Read the model definition and answer for the solid it produces. Units are mm, in the model's axes. Face numbers are marked on the shaded views. A direction names the side the tool comes from. Coordinates: 2 decimals unless noted, no trailing zeros. Write each loop counter-clockwise with the first axis right and the second up, starting at its lowest first coordinate (ties: lowest second). Pieces come first, ordered by that corner, then holes.
Item 1: Section B-B (z = 10.25) is taken. Give the vertices of the cut face in (x, y).
Item 2: A tool of negligible diameter and unlimited length cuts with its end or side. For the marked faces 1 and 2, from which of +Z, -Z, +X, -X, +Y, -Y can it reach the whole face along a straight path? Write none if from no direction.
Item 3: Each of these flat-tipped pins is pushed along its axis until it touches: P1, Ø8, axis at x = 26.5, y = -1, coming from the -Z side; P2, Ø1.4, axis at y = 0, z = 3.5, coming from the +X side; P3, Ø8, axis at x = 11.5, y = 0, coming from the +Z side; P4, Ø1.5, axis at x = 39, y = -10, coming from the +Z side. Where does it stop, or does it pass through?
Item 4: Determine the mould class of the marked faces 3, 4, 5 and 6 for opening direction Y: released by +Y, released by -Y, zero draft, split by the parting line, or undercut.
Item 5: Section A-A (y = 0) is taken. Give the vertices of the cut face in (x, z).
Item 6: Section D-D (x = -7) is taken. Give the vertices of the cut face in (y, z).
Item 7: Straight lines are drawn through the part: probe 1 along X at (y, z) = (3, 9.5); probe 2 along Y at (x, z) = (115.5, 9.25); probe 3 along Y at (x, z) = (111, 3.25). For each, find the intervals that lie inside material, in ascending order.
Item 8: Section C-C (x = 105) is taken. Give the vertices of the cut face in (y, z), then the cut area to 3 significant figures.
from build123d import *

# Parameters (mm, degrees)
F0_W         = 50.5
F0_H         = 9
F0_H_2       = 2
F0_W_2       = 12.75
F0_H_3       = 0.25
F0_W_3       = 1.2480659857
F1_DEPTH     = 1.5
F0_W_4       = 77.7519340143
F2_DEPTH     = 6.5
F3_DEPTH     = 15
F4_R         = 2
F5_DEPTH     = 162.001
F6_R         = 2
F7_T1_DEPTH  = 27.5
F7_T4_ANGLE  = 90
F7_T6_ANGLE  = 90
F7_T8_ANGLE  = 90
F7_T10_ANGLE = 90


# Not quite as in the source:
# - a fillet or chamfer that OpenCascade refuses, or shapes differently, is made with other operations: its cross-section is extruded or revolved along the edge and cut away or added


with BuildPart() as f1:
    # F0 (on Top) → F1 (new body)
    with BuildSketch(Plane.XY):
        with Locations((8.0849453807, 6.5)):
            Rectangle(F0_W, F0_H)
        with Locations((8.0849453807, 1)):
            Rectangle(F0_W, F0_H_2)
        with Locations((8.0849453807, -1)):
            Rectangle(F0_W, F0_H_2)
        with Locations((-23.5400546193, -1)):
            Rectangle(F0_W_2, F0_H_2)
        with Locations((-23.5400546193, 1)):
            Rectangle(F0_W_2, F0_H_2)
        with Locations((39.7099453807, 1)):
            Rectangle(F0_W_2, F0_H_2)
        with Locations((39.7099453807, -1)):
            Rectangle(F0_W_2, F0_H_2)
        Polygon((46.0849453807, 2), (46.0849453807, 0), (46.0849453807, -2), (123.8368793949, -2), (123.8368793949, 2), align=None)
        with Locations((8.0849453807, -6.5)):
            Rectangle(F0_W, F0_H)
        with Locations((8.0849453807, 11.125)):
            Rectangle(F0_W, F0_H_3)
        with Locations((8.0849453807, -11.125)):
            Rectangle(F0_W, F0_H_3)
        with Locations((-30.5390876122, -1)):
            Rectangle(F0_W_3, F0_H_2)
        with Locations((-30.5390876122, 1)):
            Rectangle(F0_W_3, F0_H_2)
    extrude(amount=F1_DEPTH)

    # F0 (on Top) → F2 (join)
    with BuildSketch(Plane.XY):
        with Locations((-23.5400546193, 6.5)):
            Rectangle(F0_W_2, F0_H)
        with Locations((-30.5390876122, 6.5)):
            Rectangle(F0_W_3, F0_H)
        with Locations((-23.5400546193, -6.5)):
            Rectangle(F0_W_2, F0_H)
        with Locations((-30.5390876122, -6.5)):
            Rectangle(F0_W_3, F0_H)
        with Locations((39.7099453807, -6.5)):
            Rectangle(F0_W_2, F0_H)
        with Locations((39.7099453807, 6.5)):
            Rectangle(F0_W_2, F0_H)
        with Locations((84.9609123878, 6.5)):
            Rectangle(F0_W_4, F0_H)
        with Locations((84.9609123878, -6.5)):
            Rectangle(F0_W_4, F0_H)
    extrude(amount=F2_DEPTH)

    # F0 (on Top) → F3 (join)
    with BuildSketch(Plane.XY):
        Polygon((127.3368793949, -15), (127.3368793949, 15), (-34.6631206051, 15), (-34.6631206051, 0), (-34.6631206051, -15), align=None)
        Polygon((-31.1631206051, -2), (-31.1631206051, 0), (-31.1631206051, 2), (-31.1631206051, 11), (-29.9150546193, 11), (-17.1650546193, 11), (-17.1650546193, 11.25), (33.3349453807, 11.25), (33.3349453807, 11), (46.0849453807, 11), (123.8368793949, 11), (123.8368793949, 2), (123.8368793949, -2), (123.8368793949, -11), (46.0849453807, -11), (33.3349453807, -11), (33.3349453807, -11.25), (-17.1650546193, -11.25), (-17.1650546193, -11), (-29.9150546193, -11), (-31.1631206051, -11), align=None, mode=Mode.SUBTRACT)
    extrude(amount=F3_DEPTH)

    # F4 (on face) → F5 (cut, through all)
    with BuildSketch(Plane.YZ.offset(127.3368793949)):
        with Locations((0, 4.3932246044)):
            Circle(F4_R)
    extrude(amount=-F5_DEPTH, mode=Mode.SUBTRACT)

    # F6
    f6_edges = [f1.edges().sort_by_distance(p)[0] for p in [
        (-24.164088, -2, 6.5),
        (-24.164088, 2, 6.5),
        (-17.165055, -6.5, 6.5),
        (-17.165055, 6.5, 6.5),
        (33.334945, 6.5, 6.5),
        (33.334945, -6.5, 6.5),
        (78.585912, -2, 6.5),
        (78.585912, 2, 6.5),
        (46.336879, 15, 15),
        (-34.663121, 0, 15),
        (46.336879, -15, 15),
        (127.336879, 0, 15),
    ]]
    fillet(f6_edges, radius=F6_R)

    # F7: fillet of radius 5 on 4 edges, made by hand

    # F7_s2 → F7_t1 (cut)
    with BuildSketch(Plane.XY.offset(-12.5)):
        with BuildLine():
            ThreePointArc((-29.6631206051, 15), (-33.198654511, 13.5355339059), (-34.6631206051, 10))
            Line((-34.6631206051, 10), (-34.6631206051, 15))
            Line((-34.6631206051, 15), (-29.6631206051, 15))
        make_face()
        with BuildLine():
            ThreePointArc((-34.6631206051, -10), (-33.198654511, -13.5355339059), (-29.6631206051, -15))
            Line((-29.6631206051, -15), (-34.6631206051, -15))
            Line((-34.6631206051, -15), (-34.6631206051, -10))
        make_face()
        with BuildLine():
            ThreePointArc((122.3368793949, 15), (125.8724133009, 13.5355339059), (127.3368793949, 10))
            Line((127.3368793949, 10), (127.3368793949, 15))
            Line((127.3368793949, 15), (122.3368793949, 15))
        make_face()
        with BuildLine():
            ThreePointArc((127.3368793949, -10), (125.8724133009, -13.5355339059), (122.3368793949, -15))
            Line((122.3368793949, -15), (127.3368793949, -15))
            Line((127.3368793949, -15), (127.3368793949, -10))
        make_face()
    extrude(amount=F7_T1_DEPTH, mode=Mode.SUBTRACT)

    # F7_s3 → F7_t4 (revolve, cut)
    with BuildSketch(Plane.YZ.offset(122.3368793949)):
        with BuildLine():
            ThreePointArc((-13, 15), (-14.4142135624, 14.4142135624), (-15, 13))
            Line((-15, 13), (-15, 15))
            Line((-15, 15), (-13, 15))
        make_face()
    revolve(axis=Axis((122.3368793949, -10, 15), (0, 0, 1)), revolution_arc=F7_T4_ANGLE, mode=Mode.SUBTRACT)

    # F7_s5 → F7_t6 (revolve, cut)
    with BuildSketch(Plane.XZ.offset(-10)):
        with BuildLine():
            ThreePointArc((125.3368793949, 15), (126.7510929573, 14.4142135624), (127.3368793949, 13))
            Line((127.3368793949, 13), (127.3368793949, 15))
            Line((127.3368793949, 15), (125.3368793949, 15))
        make_face()
    revolve(axis=Axis((122.3368793949, 10, 15), (0, 0, 1)), revolution_arc=F7_T6_ANGLE, mode=Mode.SUBTRACT)

    # F7_s7 → F7_t8 (revolve, cut)
    with BuildSketch(Plane.XZ.offset(10)):
        with BuildLine():
            ThreePointArc((-32.6631206051, 15), (-34.0773341674, 14.4142135624), (-34.6631206051, 13))
            Line((-34.6631206051, 13), (-34.6631206051, 15))
            Line((-34.6631206051, 15), (-32.6631206051, 15))
        make_face()
    revolve(axis=Axis((-29.6631206051, -10, 15), (0, 0, 1)), revolution_arc=F7_T8_ANGLE, mode=Mode.SUBTRACT)

    # F7_s9 → F7_t10 (revolve, cut)
    with BuildSketch(Plane.YZ.offset(-29.6631206051)):
        with BuildLine():
            ThreePointArc((13, 15), (14.4142135624, 14.4142135624), (15, 13))
            Line((15, 13), (15, 15))
            Line((15, 15), (13, 15))
        make_face()
    revolve(axis=Axis((-29.6631206051, 10, 15), (0, 0, 1)), revolution_arc=F7_T10_ANGLE, mode=Mode.SUBTRACT)


solid = f1.part
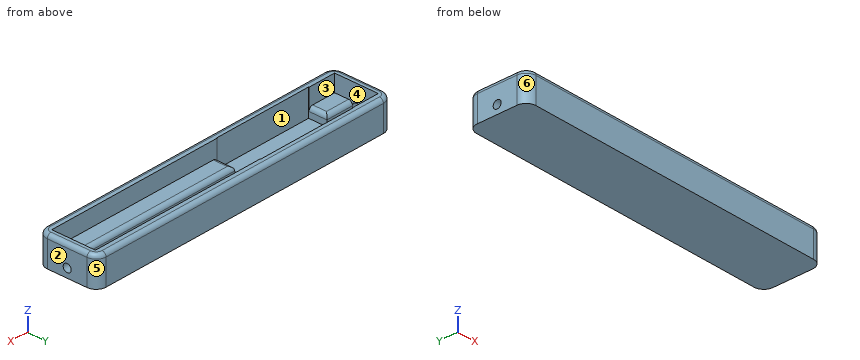
Established:
1. outline: (-34.66, -10) arc R5 ccw to (-29.66, -15) - (122.34, -15) arc R5 ccw to (127.34, -10) - (127.34, 10) arc R5 ccw to (122.34, 15) - (-29.66, 15) arc R5 ccw to (-34.66, 10) - close; hole (-31.16, -11) - (-17.17, -11) - (-17.17, -11.25) - (33.33, -11.25) - (33.33, -11) - (123.84, -11) - (123.84, 11) - (33.33, 11) - (33.33, 11.25) - (-17.17, 11.25) - (-17.17, 11) - (-31.16, 11) - close
2. face 1: +Z
2. face 2: +Z, -Z, +X, +Y, -Y
3. P1: stops at z = 0
3. P2: passes through
3. P3: stops at z = 1.5
3. P4: stops at z = 6.5
4. face 3: undercut
4. face 4: undercut
4. face 5: released by +Y
4. face 6: released by -Y
5. outline: (-34.66, 0) - (127.34, 0) - (127.34, 2.39) - (123.84, 2.39) - (123.84, 1.5) - (-31.16, 1.5) - (-31.16, 2.39) - (-34.66, 2.39) - close; (-34.66, 6.39) - (-31.16, 6.39) - (-31.16, 15) - (-32.66, 15) arc R2 ccw to (-34.66, 13) - close; (123.84, 6.39) - (127.34, 6.39) - (127.34, 13) arc R2 ccw to (125.34, 15) - (123.84, 15) - close
6. outline: (-15, 0) - (15, 0) - (15, 13) arc R2 ccw to (13, 15) - (11.25, 15) - (11.25, 1.5) - (-11.25, 1.5) - (-11.25, 15) - (-13, 15) arc R2 ccw to (-15, 13) - close
7. probe 1: x = -34.66 to -31.16, 123.84 to 127.34
7. probe 2: y = -15 to -11, 11 to 15
7. probe 3: y = -15 to -2, 2 to 15
8. outline: (-15, 0) - (15, 0) - (15, 13) arc R2 ccw to (13, 15) - (11, 15) - (11, 6.5) - (4, 6.5) arc R2 ccw to (2, 4.5) - (2, 1.5) - (-2, 1.5) - (-2, 4.5) arc R2 ccw to (-4, 6.5) - (-11, 6.5) - (-11, 15) - (-13, 15) arc R2 ccw to (-15, 13) - close
8. area: 240 mm2
